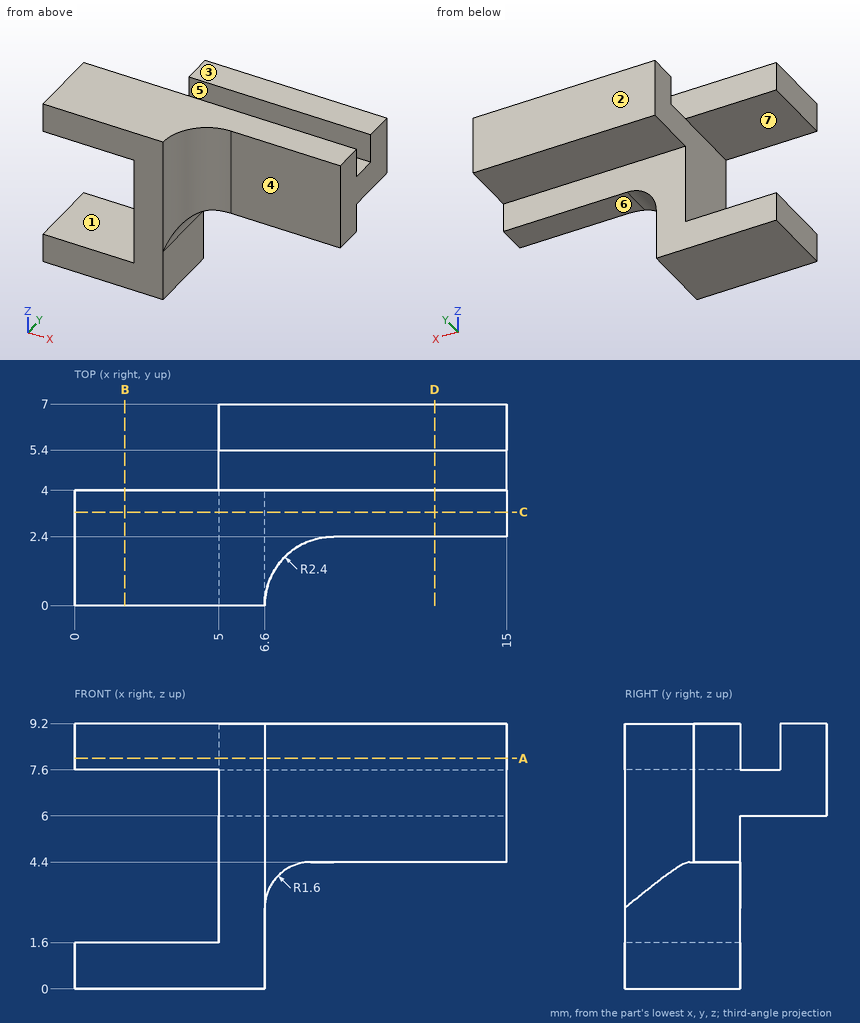
Input: dimensioned drawing with shaded views. Units: mm. Origin: part minimum x, y, z. A direction names the side the tool comes from. Round coordinates to 2 decimals unless told otherwise and drop trailing zeros. Order: outer loops, then holes, each group sorted by start corner. A loop starts at its lowest first (then second) coordinate and runs counter-clockwise, first axis right, second up.
1. Pin query (flat end, axial travel): P1, Ø3.5, axis at x = 10, y = 5, coming from the -Z side; P2, Ø3.5, axis at y = 4.5, z = 3.5, coming from the -X side; P3, Ø1.8, axis at x = 5.5, z = 4, coming from the +Y side. Return the tip coordinate at first contact, or that it passes through.
The answers:
P1: stops at z = 4.4
P2: stops at x = 5
P3: stops at y = 4
2. Cut plane C-C, the plane y = 3.25. Output: boundary loops of the cut face in (x, z).
The answers:
outline: (0, 0) - (6.6, 0) - (6.6, 2.8) arc R1.6 cw to (8.2, 4.4) - (15, 4.4) - (15, 9.2) - (0, 9.2) - (0, 7.6) - (5, 7.6) - (5, 1.6) - (0, 1.6) - close
3. Set-up query: the marked faces 4, 5, 6 and 7. Return all of +Z, -Z, +X, -X, +Y, -Y with unobstructed straight access to the full face (end or side cutting, diameter ignored); none if empty.
The answers:
face 4: +Z, -Z, +X, -Y
face 5: +Z, +X, -X
face 6: -Z, +X, +Y, -Y
face 7: -X, +Y, -Y
4. Cut plane A-A, the plane z = 8. Output: boundary loops of the cut face in (x, y), then the cut area to 3 significant figures.
The answers:
outline: (0, 0) - (6.6, 0) arc R2.4 cw to (9, 2.4) - (15, 2.4) - (15, 4) - (0, 4) - close; (5, 5.4) - (15, 5.4) - (15, 7) - (5, 7) - close
area: 57.1 mm2
5. Cut plane B-B, the plane x = 1.75. Output: boundary loops of the cut face in (y, z).
The answers:
outline: (0, 0) - (4, 0) - (4, 1.6) - (0, 1.6) - close; (0, 7.6) - (4, 7.6) - (4, 9.2) - (0, 9.2) - close
6. Mould query, pull axis Z, two halves, no side actions, for the marked faces 1, 2 and 3. Classes: released by +Z, released by -Z, zero draft, split by the parting line, or undercut.
The answers:
face 1: undercut
face 2: zero draft
face 3: released by +Z
7. Material intervals for line 1 (Z direction, x = 1.5, y = 3.25); line 2 (Y direction, x = 6.5, z = 8.5); line 3 (Y direction, x = 9.75, z = 8), sorted ascending.
The answers:
line 1: z = 0 to 1.6, 7.6 to 9.2
line 2: y = 0 to 4, 5.4 to 7
line 3: y = 2.4 to 4, 5.4 to 7
8. Cut plane D-D, the plane x = 12.5. Output: boundary loops of the cut face in (y, z), then the cut area to 3 significant figures.
The answers:
outline: (2.4, 4.4) - (4, 4.4) - (4, 6) - (7, 6) - (7, 9.2) - (5.4, 9.2) - (5.4, 7.6) - (4, 7.6) - (4, 9.2) - (2.4, 9.2) - close
area: 15.0 mm2
